Here's how the part is built. I have some questions about the finished solid (model axes, mm). Face numbers are marked on the shaded views. A direction names the side the tool comes from. Coordinates: 2 decimals unless noted, no trailing zeros. Order: outer loops, then holes, each group sorted by start corner. A loop starts at its lowest first (then second) coordinate and runs counter-clockwise, first axis right, second up. Notation, with made-up numbers: (34, -30.75) - (53, -30.75) arc R18 ccw to (53, -8.75) - close; hole circle Ø9 at (-16.5, -23). An arc over 180 degrees is marked (long way). Answer as CSV lines item,"result". Start each with the question number.
Q1. For pin 1 Ø3 at (x, z) = (-6, -2) entering from +Y (3 decimals); pin 2 Ø3 at (x, y) = (12.7, 0) entering from -Z; pin 3 Ø4.5 at (x, z) = (1, -4) entering from -Y (3 decimals), each with a flat end and sliding along its axis, tell me the tip position at first contact or that it passes through.
Q2. For the marked faces 1, 2 and 3, which set-ups out of +Z, -Z, +X, -X, +Y, -Y let a thin tool reach every point of the face, with its end or its side?
Q3. I need wall thicknesses on line 1 (X direction, y = -1.5, z = -0.75); line 2 (Y direction, x = 12.7, z = -1) (3 decimals); line 3 (Y direction, x = -12.7, z = 1.5). Which ranges of each line are inside material? Lowest first, please.
Q4. Suppose I cut it at D-D (x = -8.5). Please give me the cut outline in (y, z) (3 decimals).
Q5. Suppose I cut it at C-C (y = -4.5). Please give me the cut outline in (x, z) (3 decimals).
Q6. Suppose I cut it at B-B (x = 31.75). Please give me the cut outline in (y, z).
Q7. Suppose I cut it at A-A (z = -3.5). Count the separate pieces of the cut face and the enclosed holes in it, then the cut area to 3 significant figures.
from build123d import *

# Parameters (mm, degrees)
F0_W     = 76.2
F0_H     = 12.7
F1_DEPTH = 6.35
F4_D     = 3.4544
F6_DEPTH = 5.715
F8_D     = 4.0386
F8_DEPTH = 10.16
F8_TIP   = 1.213317848


with BuildPart() as f1:
    # F0 (on Top) → F1 (new body)
    with BuildSketch(Plane.XY):
        Rectangle(F0_W, F0_H)
    extrude(amount=F1_DEPTH)

    # F4 (through all)
    with Locations(Plane.XZ.offset(6.35)):
        with Locations((31.75, 3.175)):
            Hole(F4_D / 2)

    # F5 (on face) → F6 (join)
    with BuildSketch(Plane(origin=(0, 0, 0), x_dir=(1, 0, 0), z_dir=(0, 0, -1))):
        with BuildLine():
            ThreePointArc((-17.4625, 3.175), (-20.6375, 0), (-17.4625, -3.175))
            Line((-17.4625, -3.175), (17.4625, -3.175))
            ThreePointArc((17.4625, -3.175), (20.6375, 0), (17.4625, 3.175))
            Line((17.4625, 3.175), (-17.4625, 3.175))
        make_face()
    extrude(amount=F6_DEPTH)

    # F8
    with Locations(Plane(origin=(0, 0, -5.715), x_dir=(1, 0, 0), z_dir=(0, 0, -1))):
        with Locations((-12.7, 0), (12.7, 0)):
            Hole(F8_D / 2, depth=F8_DEPTH)
            with Locations((0, 0, -(F8_DEPTH + F8_TIP / 2))):  # 118° drill point
                Cone(0, F8_D / 2, F8_TIP, mode=Mode.SUBTRACT)


solid = f1.part
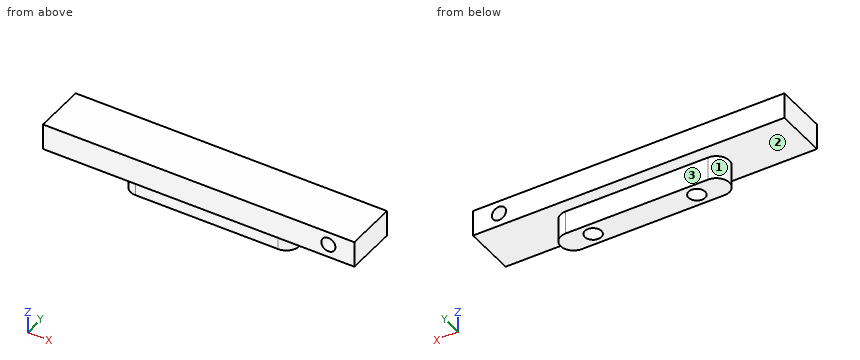
Here are the results:
1,pin 1,"stops at y = 3.175"
1,pin 2,"stops at z = 4.76"
1,pin 3,"stops at y = -3.175"
2,face 1,"-Z, -X"
2,face 2,"-Z"
2,face 3,"-Z, +X, -X, +Y"
3,line 1,"x = -20.26 to -14.05, -11.35 to 11.35, 14.05 to 20.26"
3,line 2,"y = -3.175 to -2.019, 2.019 to 3.175"
3,line 3,"y = -6.35 to -2.02, 2.02 to 6.35"
4,outline,"(-6.35, 0) - (-3.175, 0) - (-3.175, -5.715) - (3.175, -5.715) - (3.175, 0) - (6.35, 0) - (6.35, 6.35) - (-6.35, 6.35) - close"
5,outline,"(-38.1, 0) - (38.1, 0) - (38.1, 6.35) - (-38.1, 6.35) - close; hole circle Ø3.454 at (31.75, 3.175)"
6,outline,"(-6.35, 0) - (6.35, 0) - (6.35, 1.45) - (-6.35, 1.45) - close; (-6.35, 4.9) - (6.35, 4.9) - (6.35, 6.35) - (-6.35, 6.35) - close"
7,separate pieces,"1"
7,enclosed holes,"2"
7,area,"228 mm²"
